For this review, take the finished solid that the model builds, in its own axes (mm). Give positions to 0.01 mm unless a question says otherwise; leave off trailing zeros. Loops run counter-clockwise (first coordinate to the right, second up) from the corner with the lowest first, then second, coordinate; pieces in that order, holes last. Notation, with made-up numbers: M -22.5,85.5 L -13.5,85.5 A30 cw -13.5,116.5 Z; hole C 4.5,74 d4. An arc over 180 degrees is marked long. Use CSV: the item, a comma, the result in double quotes. Start each with the question number.
1. Insertion check: P1, Ø7.5, axis at x = 6, z = -9.5, coming from the +Y side; P2, Ø0.6, axis at y = 30.5, z = -11.5, coming from the -X side; P3, Ø0.9, axis at x = 29, z = -9.5, coming from the +Y side. Each pin has a flat end and moves straight along its axis. Give the tip position at first contact, or say it passes through.
2. The part is to be moulded in two halves that separate along X. For faces 1 (the face through (28.702, -13, -44)), 2 (the face through (15.56, -27.887, -30.151)), 3 (the face through (28.824, 9.077, -1.144)), 4 (the face through (-19.4, 24.2, 17.087)), say which applies: pulls with the +X half, pulls with the -X half, needs draft (parallel to the pull), parting line crosses it, or undercut.
3. Take a section at A-A, the plane z = 54. Write out the cut boundary in (x, y), and give its area (3 significant figures).
4. To check wall thickness, follow line 1 (X direction, y = 0.5, z = -24.5); line 2 (X direction, y = 0, z = -51.75). State the ranges of each line that lie inside material, in increasing order. Write a range as [from, to].
5. Take a section at B-B, the plane z = -46.5. Write out the cut boundary in (x, y), and give its area (3 significant figures).
6. Take a section at C-C, the plane y = 0. State how many separate pieces and enclosed holes the cut face has, and give its area (3 significant figures).
from build123d import *

# Parameters (mm, degrees)
F0_R      = 31.917302
F1_DEPTH  = 61.976
F2_R      = 31.934559
F3_DEPTH  = 56.388
F4_W      = 61.870079
F4_H      = 23.970603
F5_DEPTH  = 25.654
F6_W      = 34.660203
F6_H      = 23.484716
F7_DEPTH  = 55.118
F8_R      = 30.219337
F9_DEPTH  = 86.614
F10_W     = 61.384191
F10_H     = 22.350974
F11_DEPTH = 28.702
F12_W     = 25.752208
F12_H     = 21.217227
F13_DEPTH = 55.626
F14_W     = 61.222225
F14_H     = 19.111701
F15_DEPTH = 28.194
F16_W     = 62.355969
F16_H     = 19.759555
F17_DEPTH = 29.972
F18_W     = 18.949736
F18_H     = 18.787774
F19_DEPTH = 42.164
F20_W     = 26.238099
F20_H     = 18.463848
F21_DEPTH = 48.006
F22_W     = 61.870081
F22_H     = 17.087156
F23_DEPTH = 29.972
F24_W     = 61.80606
F24_H     = 17.330566
F25_DEPTH = 27.94
F26_W     = 19.759553
F26_H     = 16.925193
F27_DEPTH = 59.944
F28_W     = 27.371843
F28_H     = 17.573046
F29_DEPTH = 67.564
F30_R     = 30.730639
F31_DEPTH = 121.412
F32_W     = 61.384191
F32_H     = 17.492063
F33_DEPTH = 29.972
F34_W     = 61.041729
F34_H     = 16.627666
F35_DEPTH = 27.94
F36_W     = 27.209879
F36_H     = 15.06261
F37_DEPTH = 51.054
F38_W     = 18.62581
F38_H     = 16.52028
F39_DEPTH = 66.294
F40_W     = 60.574371
F40_H     = 23.970607
F41_DEPTH = 27.432
F42_W     = 28.18166
F42_H     = 23.160789
F43_DEPTH = 40.894
F44_W     = 60.736334
F44_H     = 23.646682
F45_DEPTH = 29.718
F46_W     = 18.949736
F46_H     = 22.512936
F47_DEPTH = 43.18


with BuildPart() as f1:
    # F0 (on Top) → F1 (new body)
    with BuildSketch(Plane.XY):
        Circle(F0_R)
    extrude(amount=F1_DEPTH)

    # F2 (on Top) → F3 (join)
    with BuildSketch(Plane.XY):
        Circle(F2_R)
    extrude(amount=-F3_DEPTH)

    # F4 (on Right) → F5 (cut)
    with BuildSketch(Plane.YZ):
        with Locations((0.08098, -38.466346)):
            Rectangle(F4_W, F4_H)
    extrude(amount=-F5_DEPTH, mode=Mode.SUBTRACT)

    # F6 (on Right) → F7 (cut)
    with BuildSketch(Plane.YZ):
        with Locations((-0.080982, -38.385364)):
            Rectangle(F6_W, F6_H)
    extrude(amount=-F7_DEPTH, mode=Mode.SUBTRACT)

    # F8 (on Top) → F9 (cut)
    with BuildSketch(Plane.XY):
        Circle(F8_R)
    extrude(amount=-F9_DEPTH, mode=Mode.SUBTRACT)

    # F10 (on Right) → F11 (cut)
    with BuildSketch(Plane.YZ):
        with Locations((0.161964, -43.487217)):
            Rectangle(F10_W, F10_H)
    extrude(amount=F11_DEPTH, mode=Mode.SUBTRACT)

    # F12 (on Right) → F13 (cut)
    with BuildSketch(Plane.YZ):
        with Locations((0.161964, -43.244272)):
            Rectangle(F12_W, F12_H)
    extrude(amount=F13_DEPTH, mode=Mode.SUBTRACT)

    # F14 (on Right) → F15 (cut)
    with BuildSketch(Plane.YZ):
        with Locations((0.080981, -12.066285)):
            Rectangle(F14_W, F14_H)
    extrude(amount=F15_DEPTH, mode=Mode.SUBTRACT)

    # F16 (on Right) → F17 (cut)
    with BuildSketch(Plane.YZ):
        with Locations((-0.161962, -11.418432)):
            Rectangle(F16_W, F16_H)
    extrude(amount=-F17_DEPTH, mode=Mode.SUBTRACT)

    # F18 (on Right) → F19 (cut)
    with BuildSketch(Plane.YZ):
        with Locations((-0.161963, -11.580395)):
            Rectangle(F18_W, F18_H)
    extrude(amount=-F19_DEPTH, mode=Mode.SUBTRACT)

    # F20 (on Right) → F21 (cut)
    with BuildSketch(Plane.YZ):
        with Locations((0.40491, -12.22825)):
            Rectangle(F20_W, F20_H)
    extrude(amount=F21_DEPTH, mode=Mode.SUBTRACT)

    # F22 (on Right) → F23 (cut)
    with BuildSketch(Plane.YZ):
        with Locations((0.080982, 8.543578)):
            Rectangle(F22_W, F22_H)
    extrude(amount=-F23_DEPTH, mode=Mode.SUBTRACT)

    # F24 (on Right) → F25 (cut)
    with BuildSketch(Plane.YZ):
        with Locations((0.210935, 8.665283)):
            Rectangle(F24_W, F24_H)
    extrude(amount=F25_DEPTH, mode=Mode.SUBTRACT)

    # F26 (on Right) → F27 (cut)
    with BuildSketch(Plane.YZ):
        with Locations((-0.080982, 8.462597)):
            Rectangle(F26_W, F26_H)
    extrude(amount=-F27_DEPTH, mode=Mode.SUBTRACT)

    # F28 (on Right) → F29 (cut)
    with BuildSketch(Plane.YZ):
        with Locations((1e-06, 8.786523)):
            Rectangle(F28_W, F28_H)
    extrude(amount=F29_DEPTH, mode=Mode.SUBTRACT)

    # F30 (on Top) → F31 (cut)
    with BuildSketch(Plane.XY):
        Circle(F30_R)
    extrude(amount=F31_DEPTH, mode=Mode.SUBTRACT)

    # F32 (on Right) → F33 (cut)
    with BuildSketch(Plane.YZ):
        with Locations((0.161964, 26.804969)):
            Rectangle(F32_W, F32_H)
    extrude(amount=-F33_DEPTH, mode=Mode.SUBTRACT)

    # F34 (on Right) → F35 (cut)
    with BuildSketch(Plane.YZ):
        with Locations((-0.009267, 27.020624)):
            Rectangle(F34_W, F34_H)
    extrude(amount=F35_DEPTH, mode=Mode.SUBTRACT)

    # F36 (on Right) → F37 (cut)
    with BuildSketch(Plane.YZ):
        with Locations((0.242946, 27.533806)):
            Rectangle(F36_W, F36_H)
    extrude(amount=F37_DEPTH, mode=Mode.SUBTRACT)

    # F38 (on Right) → F39 (cut)
    with BuildSketch(Plane.YZ):
        with Locations((0, 27.29086)):
            Rectangle(F38_W, F38_H)
    extrude(amount=-F39_DEPTH, mode=Mode.SUBTRACT)

    # F40 (on Right) → F41 (cut)
    with BuildSketch(Plane.YZ):
        with Locations((0.080981, 48.670051)):
            Rectangle(F40_W, F40_H)
    extrude(amount=F41_DEPTH, mode=Mode.SUBTRACT)

    # F42 (on Right) → F43 (cut)
    with BuildSketch(Plane.YZ):
        with Locations((0.080982, 48.912996)):
            Rectangle(F42_W, F42_H)
    extrude(amount=F43_DEPTH, mode=Mode.SUBTRACT)

    # F44 (on Right) → F45 (cut)
    with BuildSketch(Plane.YZ):
        with Locations((1e-06, 48.832014)):
            Rectangle(F44_W, F44_H)
    extrude(amount=-F45_DEPTH, mode=Mode.SUBTRACT)

    # F46 (on Right) → F47 (cut)
    with BuildSketch(Plane.YZ):
        with Locations((-0.323927, 49.074959)):
            Rectangle(F46_W, F46_H)
    extrude(amount=-F47_DEPTH, mode=Mode.SUBTRACT)


solid = f1.part
Result set:
1,P1,"y = 31.86"
1,P2,"x = 0"
1,P3,"y = 14.31"
2,face 1,"undercut"
2,face 2,"parting line crosses it"
2,face 3,"undercut"
2,face 4,"needs draft"
3,outline,"M -30.58,9.15 L -29.72,9.15 L -29.72,11.64 A31.92 ccw Z; M -30.38,-9.8 A31.92 ccw -29.72,-11.64 L -29.72,-9.8 Z; M -9.82,-30.37 A31.92 ccw 10.31,-30.21 L 5.65,-30.21 A30.73 cw -4.71,-30.37 Z; M -9.82,30.37 L -4.71,30.37 A30.73 cw 4.71,30.37 L 9.82,30.37 A31.92 ccw Z; M 27.43,-16.32 A31.92 ccw 28.68,-14.01 L 27.43,-14.01 Z; M 27.43,14.17 L 28.6,14.17 A31.92 ccw 27.43,16.32 Z"
3,area,"41.5 mm2"
4,line 1,"[-31.93, -30.22], [30.22, 31.93]"
4,line 2,"[-31.93, -30.22]"
5,outline,"M -26.88,17.25 L -25.65,17.25 L -25.65,19.02 A31.93 ccw Z; M -26.77,-17.41 A31.93 ccw -25.65,-19.02 L -25.65,-17.41 Z; M -8.24,-30.85 A31.93 ccw 9.37,-30.53 L 0,-30.53 L 0,-30.85 Z; M -7.6,31.02 L 0,31.02 L 0,30.85 L 8.24,30.85 A31.93 ccw Z; M 28.7,-14 A31.93 ccw 29.29,-12.71 L 28.7,-12.71 Z; M 28.7,13.04 L 29.15,13.04 A31.93 ccw 28.7,14 Z"
5,area,"28.0 mm2"
6,separate pieces,"12"
6,enclosed holes,"0"
6,area,"67.3 mm2"
